Part model, mm, in its own coordinate system. A direction names the side the tool comes from. Round coordinates to 2 decimals unless told otherwise and drop trailing zeros. Loops run counter-clockwise (first coordinate to the right, second up) from the corner with the lowest first, then second, coordinate; pieces in that order, holes last. Notation, with made-up numbers: (20.5, 16) - (64.5, 16) arc R30 cw to (64.5, 43) - close; hole circle Ø11 at (47, -33.5). An arc over 180 degrees is marked (long way). Put each result on its own line as item: value.
from build123d import *

# Parameters (mm, degrees)
SKETCH1_R           = 10.5
BOSS_EXTRUDE1_DEPTH = 5.5
SKETCH3_R           = 14.5
CUT_EXTRUDE1_DEPTH  = 8


with BuildPart() as part:
    # Sketch1 → Boss-Extrude1 (new, symmetric)
    with BuildSketch(Plane(origin=(0, 0, 0), x_dir=(1, 0, 0), z_dir=(0, 1, 0))):
        Polygon((6.627416998, 16), (-6.627416998, 16), (-16, 6.627416998), (-16, -6.627416998), (-6.627416998, -16), (6.627416998, -16), (16, -6.627416998), (16, 6.627416998), align=None)
        with Locations(Location((0, 0, 0), (0, 0, 270))):
            Circle(SKETCH1_R, mode=Mode.SUBTRACT)
    extrude(amount=BOSS_EXTRUDE1_DEPTH, both=True)

    # Sketch2 → Cut-Revolve1 (revolve, cut)
    with BuildSketch(Plane.XY, mode=Mode.PRIVATE) as cut_revolve1_sk:
        Polygon((-18.5, 2.1), (-18.5, 7.5), (-13.1, 7.5), align=None)
        Polygon((-13.1, -7.5), (-18.5, -2.1), (-18.5, -7.5), align=None)
    revolve(cut_revolve1_sk.sketch.rotate(Axis((0, 0, 0), (0, 1, 0)), 90), axis=Axis((0, 0, 0), (0, 1, 0)), mode=Mode.SUBTRACT)

    # Sketch3 → Cut-Extrude1 (cut)
    with BuildSketch(Plane.XZ.offset(5.5)):
        with Locations(Location((0, 0, 0), (0, 0, 270))):
            Circle(SKETCH3_R)
    extrude(amount=-CUT_EXTRUDE1_DEPTH, mode=Mode.SUBTRACT)


solid = part.part
1. Band-saw the part on C-C (x = 0). List the corners of the cut face in (y, z), plus the area to 3 significant figures.
A:
outline: (-5.5, -15.1) - (-4.6, -16) - (4.6, -16) - (5.5, -15.1) - (5.5, -10.5) - (2.5, -10.5) - (2.5, -14.5) - (-5.5, -14.5) - close; (-5.5, 14.5) - (2.5, 14.5) - (2.5, 10.5) - (5.5, 10.5) - (5.5, 15.1) - (4.6, 16) - (-4.6, 16) - (-5.5, 15.1) - close
area: 55.4 mm²
2. Tool access for faces 1 (the flat face through (11.25, 0.06, 11.38)), 2 (the flat face through (4, 2.5, -10)): list every direction of +Z, -Z, +X, -X, +Y, -Y with a clear straight run to the whole face (end or side of a thin tool).
A:
face 1: +Z, +X, +Y, -Y
face 2: -Y
3. Probe line 1 along X through (y, z) = (3.9, 0); line 2 along X through (y, z) = (-0.5, 0). List the from-to ranges inside material, lowest first. Write a range as [from, to].
A:
line 1: x = [-16, -10.5], [10.5, 16]
line 2: x = [-16, -14.5], [14.5, 16]
4. Two-plate mould, pull along X, no slides. Class faces 3 (the flat face through (11.38, 0.06, -11.25)), 4 (the conical face through (-5.837, 5.361, 14.077)), 5 (the cylindrical face through (3.2, 4, 10)), 6 (the cylindrical face through (-5.554, -1.556, -13.394)): pulls with the +X half, pulls with the -X half, needs draft (parallel to the pull), parting line crosses it, or undercut.
A:
face 3: pulls with the +X half
face 4: parting line crosses it
face 5: undercut
face 6: undercut
5. Band-saw the part on B-B (y = -1.75). List the corners of the cut face in (x, z), plus the area to 3 significant figures.
A:
outline: (-16, -6.63) - (-6.63, -16) - (6.63, -16) - (16, -6.63) - (16, 6.63) - (6.63, 16) - (-6.63, 16) - (-16, 6.63) - close; hole circle Ø29 at (0, 0)
area: 188 mm²
6. Band-saw the part on A-A (z = 0). List the corners of the cut face in (x, y), plus the area to 3 significant figures.
A:
outline: (-16, -4.6) - (-15.1, -5.5) - (-14.5, -5.5) - (-14.5, 2.5) - (-10.5, 2.5) - (-10.5, 5.5) - (-15.1, 5.5) - (-16, 4.6) - close; (10.5, 2.5) - (14.5, 2.5) - (14.5, -5.5) - (15.1, -5.5) - (16, -4.6) - (16, 4.6) - (15.1, 5.5) - (10.5, 5.5) - close
area: 55.4 mm²
7. Pin check, flat tips, straight feed: P1, Ø2, axis at x = -10.5, y = -3.5, coming from the +Z side; P2, Ø5, axis at x = -3.5, z = 10.5, coming from the -Y side. Stop position of each tip, or through.
A:
P1: stops at z = 13.13
P2: stops at y = 2.5
